The listing builds one solid part. Answer for the finished solid, in the listing's coordinates (mm). Coordinates: 2 decimals unless noted, no trailing zeros. Loops run counter-clockwise (first coordinate to the right, second up) from the corner with the lowest first, then second, coordinate; pieces in that order, holes last. Notation, with made-up numbers: M 28,16 L 78,16 A3 cw 78,20 Z; hole C 44,-33.75 d4. An arc over 180 degrees is marked long. Return JSON: item names as keys, results as strings. Group by question number.
1. Straight lines are drawn through the part: L1, parallel to Z at x = 1, y = -20.5; L2, parallel to Y at x = 0.55, z = 22; L3, parallel to Y at x = 2.85, z = 2. For each, find the intervals that lie inside material, in ascending order. Write a range as from..to.
2. Section A-A (z = 10.5) is taken. Write down the section's boundary in (x, y), then the cut area to 3 significant figures.
3. Given P1, Ø1, axis at y = -19, z = 14, coming from the -X side; P2, Ø8, axis at y = -1, z = 0.5, coming from the +X side, each flat-ended and moving along its own axis, determine where each tip first touches the part or whether it passes through.
```python
from build123d import *

# Parameters (mm, degrees)
BASPROSKE_W        = 3
BASPROSKE_H        = 24
TOOTHCUT_DEPTH     = 35.073450075
TEETHCUTS_COUNT    = 30
TEETHCUTS_ANGLE    = 348
BORSKE_R           = 2
BORE_DEPTH         = 50.001016
CUT_EXTRUDE1_DEPTH = 35.010864624


with BuildPart() as part:
    # BasProSke → Base-Revolve (revolve)
    with BuildSketch(Plane(origin=(0, 0, 0), x_dir=(1, 0, 0), z_dir=(0, 1, 0)), mode=Mode.PRIVATE) as base_revolve_sk:
        with Locations((1.5, 12)):
            Rectangle(BASPROSKE_W, BASPROSKE_H)
    revolve(base_revolve_sk.sketch.rotate(Axis((-10, 0, 0), (1, 0, 0)), 180), axis=Axis((-10, 0, 0), (1, 0, 0)))

    # TooCutSke → ToothCut (cut, through all)
    with BuildSketch(Plane(origin=(0, 0, 0), x_dir=(0, 0, -1), z_dir=(1, 0, 0))):
        with BuildLine():
            ThreePointArc((0.693278797, 20.612344372), (0, 20.624), (-0.693278797, 20.612344372))
            ThreePointArc((-0.693278797, 20.612344372), (-1.270739341, 22.465148834), (-2.231973449, 24.151083009))
            ThreePointArc((-2.231973449, 24.151083009), (0, 24.254), (2.231973449, 24.151083009))
            ThreePointArc((2.231973449, 24.151083009), (1.270739341, 22.465148834), (0.693278797, 20.612344372))
        make_face()
    toothcut = extrude(amount=TOOTHCUT_DEPTH, mode=Mode.SUBTRACT)

    # TeethCuts: ToothCut ×30 about axis
    teethcuts_axis = Axis((-10, 0, 0), (1, 0, 0))
    for i in range(1, TEETHCUTS_COUNT):
        add(toothcut.rotate(teethcuts_axis, i * TEETHCUTS_ANGLE / (TEETHCUTS_COUNT - 1)), mode=Mode.SUBTRACT)

    # BorSke → Bore (cut, symmetric)
    with BuildSketch(Plane(origin=(0, 0, 0), x_dir=(0, 0, -1), z_dir=(1, 0, 0))):
        with Locations(Location((0, 0, 0), (0, 0, 180))):
            Circle(BORSKE_R)
    extrude(amount=BORE_DEPTH, both=True, mode=Mode.SUBTRACT)

    # Sketch2 → Cut-Extrude1 (cut, through all)
    with BuildSketch(Plane.ZY):
        with BuildLine():
            Line((-1.88348082, 2.95), (-15.34156858, 1.994983292))
            ThreePointArc((-15.34156858, 1.994983292), (-17.2, 0), (-15.34156858, -1.994983292))
            Line((-15.34156858, -1.994983292), (-1.88348082, -2.95))
            ThreePointArc((-1.88348082, -2.95), (0, -3.5), (1.88348082, -2.95))
            Line((1.88348082, -2.95), (15.34156858, -1.994983292))
            ThreePointArc((15.34156858, -1.994983292), (17.2, 0), (15.34156858, 1.994983292))
            Line((15.34156858, 1.994983292), (1.88348082, 2.95))
            ThreePointArc((1.88348082, 2.95), (0, 3.5), (-1.88348082, 2.95))
        make_face()
    extrude(amount=-CUT_EXTRUDE1_DEPTH, mode=Mode.SUBTRACT)


solid = part.part
```
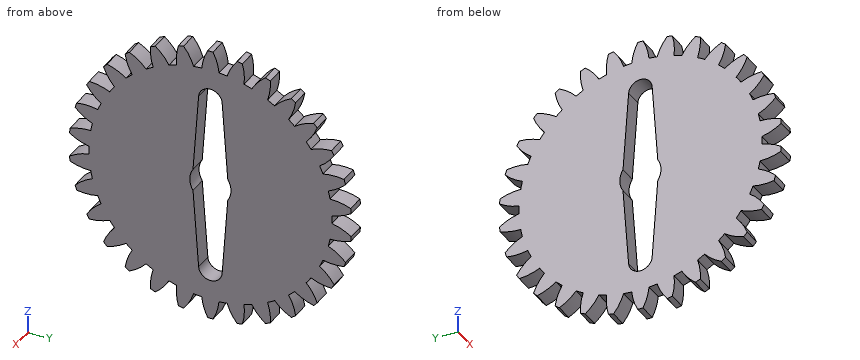
Worked out:
{
 "1": {"L1": "-12.38..-10.89, -7.96..-5.19, -3.61..3.61, 5.19..7.96, 10.89..12.38", "L2": "-9.59..-9.22, -5.71..-3.5, -1.22..1.22, 3.5..5.71, 9.22..9.59", "L3": "-23.81..-2.94, 2.94..23.81"},
 "2": {"outline": "M 0,-20.19 L 3,-20.19 L 3,-2.34 L 0,-2.34 Z; M 0,2.34 L 3,2.34 L 3,20.19 L 0,20.19 Z", "area": "107 mm^2"},
 "3": {"P1": "through", "P2": "x = 3"}
}
